CAD build for the part. Positions are in the model's coordinates, mm. Face numbers are marked on the shaded views. A direction names the side the tool comes from. Round coordinates to 2 decimals unless told otherwise and drop trailing zeros. Loops run counter-clockwise (first coordinate to the right, second up) from the corner with the lowest first, then second, coordinate; pieces in that order, holes last.
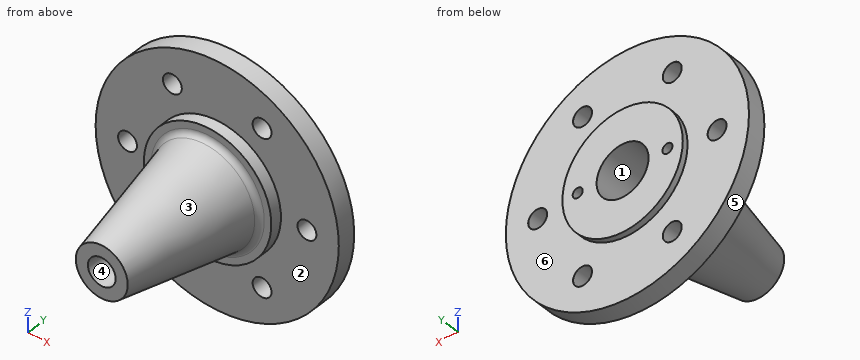
from build123d import *

# Parameters (mm, degrees)
FILLET1_R                            = 5
F_16_0_16_DIAMETER_HOLE1_D           = 16
F_16_0_16_DIAMETER_HOLE1_CSINK_D     = 16.05
F_16_0_16_DIAMETER_HOLE1_CSINK_ANGLE = 90
CIRPATTERN1_COUNT                    = 6
M10X1_5_TAPPED_HOLE1_D               = 8.5
M10X1_5_TAPPED_HOLE1_DEPTH           = 18
M10X1_5_TAPPED_HOLE1_TIP             = 2.553657631


with BuildPart() as part:
    # Sketch1 → Revolve1 (revolve)
    with BuildSketch(Plane.XY, mode=Mode.PRIVATE) as revolve1_sk:
        Polygon((0, 0), (51, 0), (51, -5), (103, -5), (103, -21), (54, -21), (54, -31), (44, -31), (22, -141), (0, -141), align=None)
    revolve(revolve1_sk.sketch.rotate(Axis((0, 0, 0), (0, -1, 0)), 180), axis=Axis((0, 0, 0), (0, -1, 0)))

    # Sketch2 → Cut-Revolve1 (revolve, cut)
    with BuildSketch(Plane.XY):
        Polygon((-11.75, -141), (-11.75, -103), (-16, -100.240017729), (-16, -86.247037966), (-11, -83), (-11, -51.143483525), (-22, -44), (-22, 0), (0, 0), (0, -141), align=None)
    revolve(axis=Axis((0, 0, 0), (0, -1, 0)), mode=Mode.SUBTRACT)

    # Fillet1
    fillet1_edges = [part.edges().sort_by_distance(p)[0] for p in [
        (44, -31, 0),
    ]]
    fillet(fillet1_edges, radius=FILLET1_R)

    # Ø16.0 (16) Diameter Hole1 (through all)
    with Locations(Plane(origin=(0, -5, 0), x_dir=(1, 0, 0), z_dir=(0, 1, 0))):
        with Locations((-76, 0)):
            f_16_0_16_diameter_hole1 = CounterSinkHole(F_16_0_16_DIAMETER_HOLE1_D / 2, F_16_0_16_DIAMETER_HOLE1_CSINK_D / 2, counter_sink_angle=F_16_0_16_DIAMETER_HOLE1_CSINK_ANGLE)

    # CirPattern1: Ø16.0 (16) Diameter Hole1 ×6 about axis
    cirpattern1_axis = Axis((0, 0, 0), (0, 1, 0))
    for i in range(1, CIRPATTERN1_COUNT):
        add(f_16_0_16_diameter_hole1.rotate(cirpattern1_axis, i * 360 / CIRPATTERN1_COUNT), mode=Mode.SUBTRACT)

    # M10x1.5 Tapped Hole1
    with Locations(Plane(origin=(0, 0, 0), x_dir=(1, 0, 0), z_dir=(0, 1, 0))):
        with Locations((38, 0), (-38, 0)):
            Hole(M10X1_5_TAPPED_HOLE1_D / 2, depth=M10X1_5_TAPPED_HOLE1_DEPTH)
            with Locations((0, 0, -(M10X1_5_TAPPED_HOLE1_DEPTH + M10X1_5_TAPPED_HOLE1_TIP / 2))):  # 118° drill point
                Cone(0, M10X1_5_TAPPED_HOLE1_D / 2, M10X1_5_TAPPED_HOLE1_TIP, mode=Mode.SUBTRACT)


solid = part.part
Item 1: Cut at B-B (y = -57). List the corners of the cut face in (x, z).
Verdict:
outline: circle Ø77.6 at (0, 0); hole circle Ø22 at (0, 0)
Item 2: Mould opens along Z. For the marked faces 1, 2, 3 and 4 say: released by +Z, released by -Z, zero draft, split by the parting line, or undercut.
Verdict:
face 1: undercut
face 2: zero draft
face 3: split by the parting line
face 4: undercut
Item 3: Cut at C-C (x = -76). List the corners of the cut face in (y, z) (3 decimals), plus the area to 3 significant figures.
Verdict:
outline: (-21, -69.52) - (-5, -69.52) - (-5, -8.025) - (-5.025, -8) - (-21, -8) - close; (-21, 8) - (-5.025, 8) - (-5, 8.025) - (-5, 69.52) - (-21, 69.52) - close
area: 1,970 mm2
Item 4: Flat gauge pins, fed straight in: P1, Ø11, axis at x = 38, z = 0, coming from the +Y side; P2, Ø12, axis at x = 73, z = 0, coming from the +Y side; P3, Ø12, axis at x = -5.5, y = -86.5, coming from the +Z side; P4, Ø10, axis at y = -58.5, z = -38, coming from the -X side. Where does each tip first touch, or does it go through?
Verdict:
P1: stops at y = 0
P2: stops at y = -5
P3: stops at z = 33.86
P4: stops at x = -20.05
Item 5: Cut at D-D (z = 85.5). List the corners of the cut face in (x, y).
Verdict:
outline: (-57.43, -21) - (57.43, -21) - (57.43, -5) - (-57.43, -5) - close
Item 6: 3-axis set-ups, long thin cutter, end or side, ignore diameter. For the marked faces 5 and 6: which of +Z, -Z, +X, -X, +Y, -Y reach the whole face in a straight line?
Verdict:
face 5: +Y, -Y
face 6: +Y
Item 7: Wall check: L1, parallel to Z at x = 38, y = -13; L2, parallel to Z at x = -43, y = -13; L3, parallel to Z at x = 76, y = -16.25. Give the ranges that are in metal, low to high.
Verdict:
L1: z = -95.73 to -73.82, -57.82 to -4.25, 4.25 to 57.82, 73.82 to 95.73
L2: z = -93.59 to -72.06, -59.57 to 59.57, 72.06 to 93.59
L3: z = -69.52 to -8, 8 to 69.52
